```python
from build123d import *

# Parameters (mm, degrees)
F0_W     = 32
F0_H     = 46
F0_W_2   = 8
F0_H_2   = 40
F0_R     = 2
F1_DEPTH = 4
F2_W     = 4
F2_H     = 2
F2_H_2   = 4
F3_DEPTH = 8
F4_W     = 4
F4_H     = 22
F5_DEPTH = 4


with BuildPart() as f1:
    # F0 (on Front) → F1 (new body)
    with BuildSketch(Plane.XZ):
        with Locations((0, -23)):
            Rectangle(F0_W, F0_H)
        with Locations((-8, -24)):
            Rectangle(F0_W_2, F0_H_2, mode=Mode.SUBTRACT)
        with Locations((0, -40)):
            Circle(F0_R, mode=Mode.SUBTRACT)
        with Locations((0, -27)):
            Circle(F0_R, mode=Mode.SUBTRACT)
        with Locations((8, -24)):
            Rectangle(F0_W_2, F0_H_2, mode=Mode.SUBTRACT)
        with Locations((0, -12)):
            Circle(F0_R, mode=Mode.SUBTRACT)
    extrude(amount=F1_DEPTH)

    # F2 (on face) → F3 (join)
    with BuildSketch(Plane(origin=(0, 0, 0), x_dir=(-1, 0, 0), z_dir=(0, 1, 0))):
        with Locations((-14, -45)):
            Rectangle(F2_W, F2_H)
        with Locations((14, -45)):
            Rectangle(F2_W, F2_H)
        with Locations((-14, -2)):
            Rectangle(F2_W, F2_H_2)
        with Locations((14, -2)):
            Rectangle(F2_W, F2_H_2)
        with Locations((0, -2)):
            Rectangle(F2_W, F2_H_2)
        with Locations((-14, -26)):
            Rectangle(F2_W, F2_H_2)
        with Locations((14, -26)):
            Rectangle(F2_W, F2_H_2)
    extrude(amount=F3_DEPTH)

    # F4 (on face) → F5 (join)
    with BuildSketch(Plane(origin=(0, 8, 0), x_dir=(-1, 0, 0), z_dir=(0, 1, 0))):
        with Locations((-14, -35)):
            Rectangle(F4_W, F4_H)
        with Locations((14, -35)):
            Rectangle(F4_W, F4_H)
    extrude(amount=-F5_DEPTH)


solid = f1.part
```
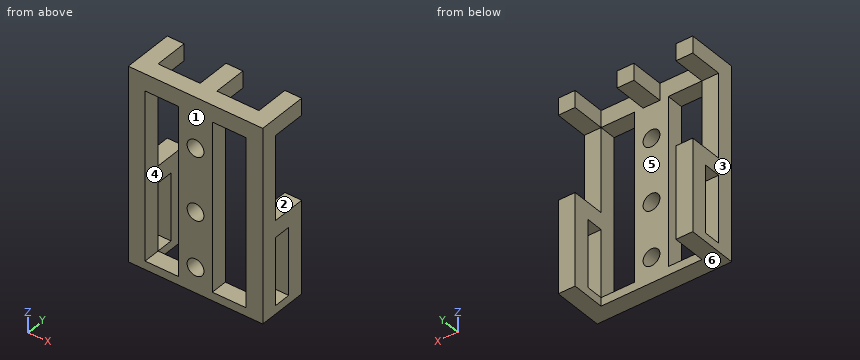
Geometry: final body of the model. Coordinates: model frame, mm. Face numbers are marked on the shaded views. A direction names the side the tool comes from. Give positions to 0.01 mm unless a question says otherwise; leave off trailing zeros. Loops run counter-clockwise (first coordinate to the right, second up) from the corner with the lowest first, then second, coordinate; pieces in that order, holes last. Notation, with made-up numbers: (21.25, 58) -> (76.25, 58) arc R30 ccw to (76.25, 86) -> close; hole circle Ø1 at (17, 62.25). An arc over 180 degrees is marked (long way). Use one line per item in the form item = value.
Item 1: Section query A-A on y = 3. Output: boundary loops of the cut face in (x, z).
A:
outline = (-16, -46) -> (-12, -46) -> (-12, -44) -> (-16, -44) -> close; (-16, -28) -> (-12, -28) -> (-12, -24) -> (-16, -24) -> close; (-16, -4) -> (-12, -4) -> (-12, 0) -> (-16, 0) -> close; (-2, -4) -> (2, -4) -> (2, 0) -> (-2, 0) -> close; (12, -46) -> (16, -46) -> (16, -44) -> (12, -44) -> close; (12, -28) -> (16, -28) -> (16, -24) -> (12, -24) -> close; (12, -4) -> (16, -4) -> (16, 0) -> (12, 0) -> close
Item 2: Line query: probe 1 along Z at (x, y) = (0, -3.05); probe 2 along Z at (x, y) = (14.5, 1.5); probe 3 along X at (y, z) = (-0.5, -6). Output: solid intervals per line, ascending.
A:
probe_1 = -46 to -42, -38 to -29, -25 to -14, -10 to 0
probe_2 = -46 to -44, -28 to -24, -4 to 0
probe_3 = -16 to -12, -4 to 4, 12 to 16
Item 3: Draft query along X for the marked faces 3, 4, 5 and 6. Return one class per face: pulls with the +X half, pulls with the -X half, needs draft (parallel to the pull), parting line crosses it, or undercut.
A:
face_3 = pulls with the -X half
face_4 = undercut
face_5 = undercut
face_6 = needs draft
Item 4: Section query D-D on z = -36. Output: boundary loops of the cut face in (x, y).
A:
outline = (-16, -4) -> (-12, -4) -> (-12, 0) -> (-16, 0) -> close; (-16, 4) -> (-12, 4) -> (-12, 8) -> (-16, 8) -> close; (-4, -4) -> (4, -4) -> (4, 0) -> (-4, 0) -> close; (12, -4) -> (16, -4) -> (16, 0) -> (12, 0) -> close; (12, 4) -> (16, 4) -> (16, 8) -> (12, 8) -> close
Item 5: Section query C-C on x = -5. Output: boundary loops of the cut face in (y, z).
A:
outline = (-4, -46) -> (0, -46) -> (0, -44) -> (-4, -44) -> close; (-4, -4) -> (0, -4) -> (0, 0) -> (-4, 0) -> close
Item 6: Pin query (flat end, axial travel): P1, Ø1, axis at x = 1.5, z = -41, coming from the +Y side. Return the tip coordinate at first contact, or that it passes through.
A:
P1 = 0
Item 7: Access query for the marked faces 1 and 2. Directions: +Z, -Z, +X, -X, +Y, -Y. A direction counts if a zero-diameter tool reaches every point of the face in a straight line with its end or side. Return the directions, or none.
A:
face_1 = +Z, -Z, +X, -X, -Y
face_2 = +X, -X, +Y
Item 8: Section query B-B on z = -12. Output: boundary loops of the cut face in (x, y).
A:
outline = (-16, -4) -> (-12, -4) -> (-12, 0) -> (-16, 0) -> close; (-4, -4) -> (-2, -4) -> (-2, 0) -> (-4, 0) -> close; (2, -4) -> (4, -4) -> (4, 0) -> (2, 0) -> close; (12, -4) -> (16, -4) -> (16, 0) -> (12, 0) -> close
